Check sheet for the drawn part. Datum: minimum x, y, z corner. Units: mm. Round coordinates to 2 decimals unless told otherwise and drop trailing zeros. Write each loop counter-clockwise with the first axis right and the second up, starting at its lowest first coordinate (ties: lowest second). Pieces come first, ordered by that corner, then holes. Notation, with made-up numbers: (48, -24) -> (57, -24) arc R22 cw to (57, -4) -> close; hole circle Ø4 at (-3.5, 17.5). An arc over 180 degrees is marked (long way). One line per item, written item: value.
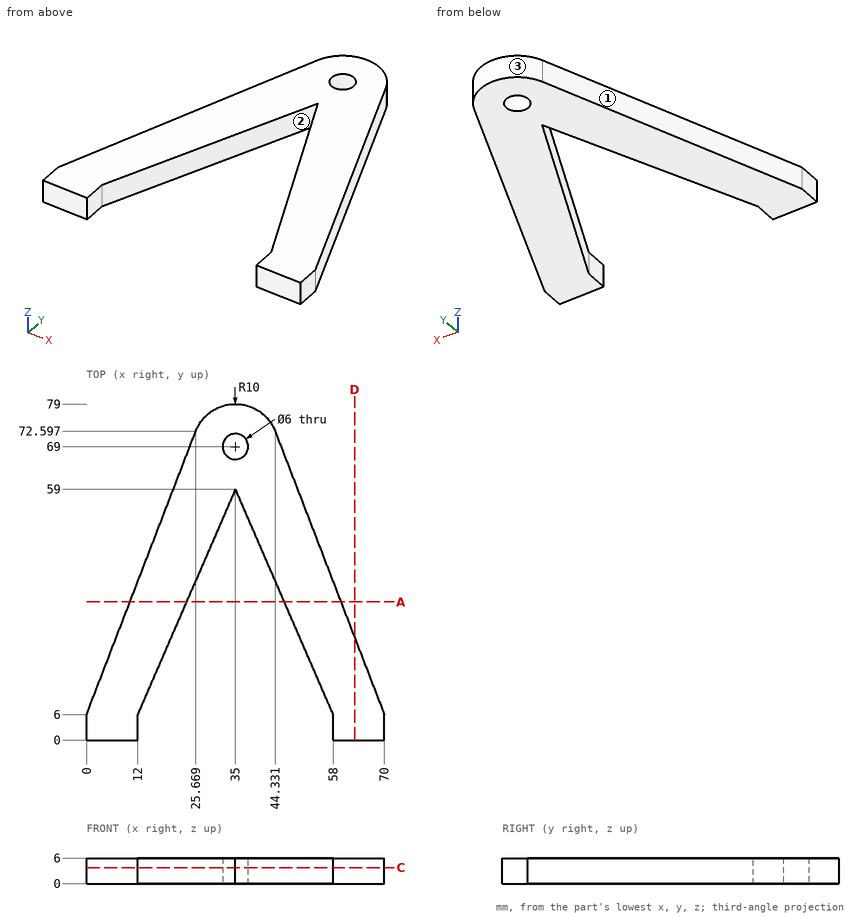
Item 1: Thickness scan on line 1 (X direction, y = 27, z = 0.95) (1 decimal); line 2 (X direction, y = 5, z = 4.25); line 3 (Y direction, x = 41, z = 4.25) (1 decimal). Record the ranges inside material, lowest first.
Answer:
line 1: x = 8.1 to 21.1, 48.9 to 61.9
line 2: x = 0 to 12, 58 to 70
line 3: y = 45.2 to 77
Item 2: Mould release check, pull along X, two halves, no side actions. Record for the marked faces 1, 2 and 3: pulls with the +X half, pulls with the -X half, needs draft (parallel to the pull), parting line crosses it, or undercut.
Answer:
face 1: pulls with the -X half
face 2: undercut
face 3: parting line crosses it
Item 3: Depth check by flat-ended pin: P1, Ø1.5, axis at y = 9, z = 2.5, coming from the -X side; P2, Ø2, axis at y = 30, z = 5, coming from the +X side (1 decimal); P3, Ø1.5, axis at x = 25.5, z = 2, coming from the -Y side. Enter the tip coordinate at first touch or a pass-through.
Answer:
P1: stops at x = 0.87
P2: stops at x = 61.1
P3: stops at y = 35.38
Item 4: Sectioned sample at A-A on y = 32.5. Enter the section's corners in (x, z) (1 decimal).
Answer:
outline: (10.2, 0) -> (23.5, 0) -> (23.5, 6) -> (10.2, 6) -> close; (46.5, 0) -> (59.8, 0) -> (59.8, 6) -> (46.5, 6) -> close
Item 5: Sectioned sample at D-D on x = 63. Enter the section's corners in (y, z), and give its area (3 significant figures).
Answer:
outline: (0, 0) -> (24.16, 0) -> (24.16, 6) -> (0, 6) -> close
area: 145 mm^2
Item 6: Sectioned sample at C-C on z = 3.75. Enter the section's corners in (x, y), and give its area (3 significant figures).
Answer:
outline: (0, 0) -> (12, 0) -> (12, 6) -> (35, 59) -> (58, 6) -> (58, 0) -> (70, 0) -> (70, 6) -> (44.33, 72.6) arc R10 ccw to (25.67, 72.6) -> (0, 6) -> close; hole circle Ø6 at (35, 69)
area: 1,940 mm^2
